Work out the finished part from the listing and answer in its coordinate system (mm). Give positions to 0.01 mm unless a question says otherwise; leave off trailing zeros. Loops run counter-clockwise (first coordinate to the right, second up) from the corner with the lowest first, then second, coordinate; pieces in that order, holes last. Notation, with made-up numbers: (83, 26) - (111, 26) arc R15 cw to (111, 48) - close; hole circle Ø11 at (89, -7.5). An arc over 180 degrees is marked (long way). Use CSV: the item, a comma, the result in double quotes.
from build123d import *

# Parameters (mm, degrees)
ESBO_O1_W                = 50
ESBO_O1_H                = 7
ESBO_O1_R                = 1
ESBO_O1_R_2              = 2.25
RESSALTO_EXTRUS_O1_DEPTH = 5
FILETE1_R                = 3.5


with BuildPart() as part:
    # Esboço1 → Ressalto-extrusão1 (new body)
    with BuildSketch(Plane.XY):
        with Locations((25, 3.5)):
            Rectangle(ESBO_O1_W, ESBO_O1_H)
        with Locations((25, 3.5)):
            Circle(ESBO_O1_R, mode=Mode.SUBTRACT)
        with Locations((4, 3.5)):
            Circle(ESBO_O1_R_2, mode=Mode.SUBTRACT)
        with Locations((46, 3.5)):
            Circle(ESBO_O1_R_2, mode=Mode.SUBTRACT)
    extrude(amount=RESSALTO_EXTRUS_O1_DEPTH)

    # Filete1
    filete1_edges = [part.edges().sort_by_distance(p)[0] for p in [
        (50, 0, 2.5),
        (50, 7, 2.5),
        (0, 0, 2.5),
        (0, 7, 2.5),
    ]]
    fillet(filete1_edges, radius=FILETE1_R - 0.0001)  # a hair under: the kernel refuses the full size


solid = part.part
Item 1: A cutting plane is placed at B-B on y = 3. Determine the outline of the cut face in (x, z).
Determined:
outline,"(0.04, 0) - (1.81, 0) - (1.81, 5) - (0.04, 5) - close; (6.19, 0) - (24.13, 0) - (24.13, 5) - (6.19, 5) - close; (25.87, 0) - (43.81, 0) - (43.81, 5) - (25.87, 5) - close; (48.19, 0) - (49.96, 0) - (49.96, 5) - (48.19, 5) - close"
Item 2: A cutting plane is placed at D-D on x = 4. Determine the outline of the cut face in (y, z), and give its area (3 significant figures).
Determined:
outline,"(0, 0) - (1.25, 0) - (1.25, 5) - (0, 5) - close; (5.75, 0) - (7, 0) - (7, 5) - (5.75, 5) - close"
area,"12.5 mm²"
Item 3: Given P1, Ø1, axis at y = 1.5, z = 1.5, coming from the +X side; P2, Ø4, axis at x = 4, y = 3.5, coming from the -Z side; P3, Ø2, axis at y = 1.5, z = 1, coming from the +X side, each flat-ended and moving along its own axis, determine where each tip first touches the part or whether it passes through.
Determined:
P1,"stops at x = 49.66"
P2,"passes through"
P3,"stops at x = 49.85"
Item 4: A cutting plane is placed at A-A on x = 25. Determine the outline of the cut face in (y, z), and give its area (3 significant figures).
Determined:
outline,"(0, 0) - (2.5, 0) - (2.5, 5) - (0, 5) - close; (4.5, 0) - (7, 0) - (7, 5) - (4.5, 5) - close"
area,"25.0 mm²"
Item 5: A cutting plane is placed at C-C on z = 2.1. State how many separate pieces and enclosed holes the cut face has, and give its area (3 significant figures).
Determined:
separate pieces,"1"
enclosed holes,"3"
area,"305 mm²"
Item 6: The mould has two halves that part along Y. Classify faces 1 (the flat face through (25, 5, 0)), 2 (the cylindrical face through (43.752, 3.599, 2.465)), 3 (the flat face through (25, 0, 2)): pulls with the +Y half, pulls with the -Y half, needs draft (parallel to the pull), parting line crosses it, or undercut.
Determined:
face 1,"needs draft"
face 2,"undercut"
face 3,"pulls with the -Y half"
Item 7: Find the intervals of material crossed by line 1 (Y direction, x = 4, z = 3.95); line 2 (X direction, y = 4, z = 4.1); line 3 (X direction, y = 5, z = 2.7), in increasing order.
Determined:
line 1,"y = 0 to 1.25, 5.75 to 7"
line 2,"x = 0.04 to 1.81, 6.19 to 24.13, 25.87 to 43.81, 48.19 to 49.96"
line 3,"x = 0.34 to 2.32, 5.68 to 44.32, 47.68 to 49.66"
